from build123d import *

# Parameters (mm, degrees)
SKETCH1_R           = 38.3
SKETCH1_R_2         = 21
BOSS_EXTRUDE1_DEPTH = 4
CUT_EXTRUDE1_DEPTH  = 10


with BuildPart() as part:
    # Sketch1 → Boss-Extrude1 (new body)
    with BuildSketch(Plane(origin=(0, 0, 0), x_dir=(1, 0, 0), z_dir=(0, 1, 0))):
        with Locations(Location((0, 0, 0), (0, 0, 270))):
            Circle(SKETCH1_R)
        with Locations(Location((0, 0, 0), (0, 0, 270))):
            Circle(SKETCH1_R_2, mode=Mode.SUBTRACT)
        Polygon((12.4, -27.481872813), (15, -28.982983513), (17.6, -27.481872813), (17.6, -24.479651414), (15, -22.978540714), (12.4, -24.479651414), align=None, mode=Mode.SUBTRACT)
        Polygon((30, 3.0022214), (27.4, 1.5011107), (27.4, -1.5011107), (30, -3.0022214), (32.6, -1.5011107), (32.6, 1.5011107), align=None, mode=Mode.SUBTRACT)
        Polygon((-17.6, -24.479651414), (-17.6, -27.481872813), (-15, -28.982983513), (-12.4, -27.481872813), (-12.4, -24.479651414), (-15, -22.978540714), align=None, mode=Mode.SUBTRACT)
        Polygon((-30, 3.0022214), (-32.6, 1.5011107), (-32.6, -1.5011107), (-30, -3.0022214), (-27.4, -1.5011107), (-27.4, 1.5011107), align=None, mode=Mode.SUBTRACT)
        Polygon((-12.4, 27.481872813), (-15, 28.982983513), (-17.6, 27.481872813), (-17.6, 24.479651414), (-15, 22.978540714), (-12.4, 24.479651414), align=None, mode=Mode.SUBTRACT)
        Polygon((17.6, 24.479651414), (17.6, 27.481872813), (15, 28.982983513), (12.4, 27.481872813), (12.4, 24.479651414), (15, 22.978540714), align=None, mode=Mode.SUBTRACT)
    extrude(amount=BOSS_EXTRUDE1_DEPTH)

    # Sketch2 → Cut-Extrude1 (cut)
    with BuildSketch(Plane(origin=(0, 4, 0), x_dir=(1, 0, 0), z_dir=(0, 1, 0))):
        with BuildLine():
            Line((6, 50.276302336), (6, 14.297506921))
            ThreePointArc((6, 14.297506921), (13.428105902, 7.752720557), (15.382004204, -1.952601038))
            Line((15.382004204, -1.952601038), (46.540555031, -19.941998745))
            ThreePointArc((46.540555031, -19.941998745), (-43.84951462, -25.31652907), (6, 50.276302336))
        make_face()
    extrude(amount=-CUT_EXTRUDE1_DEPTH, mode=Mode.SUBTRACT)


solid = part.part
Build history of the part. All positions in model axes, mm. A direction names the side the tool comes from. Coordinates: 2 decimals unless noted, no trailing zeros. Order: outer loops, then holes, each group sorted by start corner. A loop starts at its lowest first (then second) coordinate and runs counter-clockwise, first axis right, second up. Notation, with made-up numbers: M -31,-13.75 L -27,-13.75 A13 ccw -27,9.25 Z; hole C -36,68 d11. An arc over 180 degrees is marked long. One line per question, with ' | ' between items. Start each with the question number.
Q1. 3-axis set-ups, long thin cutter, end or side, ignore diameter. For faces 5 (the face through (12.4, 2, -26)), 6 (the face through (6, 2, -29)): which of +Z, -Z, +X, -X, +Y, -Y reach the whole face in a straight line?
Q2. Saw through at B-B (z = -25). List the corners of the cut face in (x, y).
Q3. Saw through at C-C (y = 1.55). List the corners of the cut face in (x, z).
Q4. Two-plate mould, pull along X, no slides. Class faces 1 (the face through (27.99, 2.03, 9.23)), 2 (the face through (31.282, 1.972, 2.262)), 3 (the face through (22, 4, -12)), 4 (the face through (17.6, 2, -26)): +X half, -X half, draft (parallel to the pull), parting line (faces both ways), or undercut.
Q5. Flat gauge pins, fed straight in: pin 1 Ø1.5 at (y, z) = (1.5, -0.5) entering from -X; pin 2 Ø0.9 at (y, z) = (1, -0.5) entering from +X. Where does each tip first touch, or does it go through?
Q6. Probe L1, parallel to X at y = 2.95, z = 2; L2, parallel to Z at x = 14.5, y = 2.9; L3, parallel to X at y = 2.6, z = -24. List the from-to ranges inside material, lowest first. Write a range as from..to.
Q7. Saw through at D-D (x = 23). List the corners of the cut face in (y, z).
Q8. Saw through at A-A (x = 29). List the corners of the cut face in (y, z).
Check values:
1) face 5: +Y, -Y | face 6: +Z, -Z, -X, +Y, -Y
2) outline: M 6,0 L 12.4,0 L 12.4,4 L 6,4 Z; M 17.6,0 L 29.02,0 L 29.02,4 L 17.6,4 Z
3) outline: M 6,-37.83 A38.3 ccw 35.76,13.72 L 20.43,4.87 A21 cw 6,-20.12 Z; hole M 12.4,-27.48 L 15,-28.98 L 17.6,-27.48 L 17.6,-24.48 L 15,-22.98 L 12.4,-24.48 Z; hole M 27.4,-1.5 L 30,-3 L 32.6,-1.5 L 32.6,1.5 L 30,3 L 27.4,1.5 Z
4) face 1: -X half | face 2: undercut | face 3: draft | face 4: undercut
5) pin 1: stops at x = 20.96 | pin 2: stops at x = 38.3
6) L1: x = 20.9..28.26, 31.74..38.25 | L2: z = -35.45..-28.69, -23.27..-15.19 | L3: x = 6..13.23, 16.77..29.85
7) outline: M 0,-30.62 L 4,-30.62 L 4,6.35 L 0,6.35 Z
8) outline: M 0,-25.02 L 4,-25.02 L 4,-2.42 L 0,-2.42 Z; M 0,2.42 L 4,2.42 L 4,9.81 L 0,9.81 Z
